from build123d import *

# Parameters (mm, degrees)
F0_R     = 4.8895
F1_DEPTH = 1.5875
F2_R     = 5.08
F3_R     = 5.08
F4_R     = 6.35
F5_R     = 5.08
F7_DEPTH = 12.7
F8_R     = 6.1595
F9_DEPTH = 1.5875
F10_R    = 0.635


with BuildPart() as f1:
    # F0 (on Right) → F1 (new body, symmetric)
    with BuildSketch(Plane.YZ):
        with BuildLine():
            Line((15.980706, -19.05), (23.759998, -9.779))
            ThreePointArc((23.759998, -9.779), (33.538998, 0), (23.759998, 9.779))
            Line((23.759998, 9.779), (15.875, 9.779))
            Line((15.875, 9.779), (10.546717, 3.429))
            Line((10.546717, 3.429), (-10.546717, 3.429))
            Line((-10.546717, 3.429), (-15.875, 9.779))
            Line((-15.875, 9.779), (-23.759998, 9.779))
            ThreePointArc((-23.759998, 9.779), (-33.538998, 0), (-23.759998, -9.779))
            Line((-23.759998, -9.779), (-15.980706, -19.05))
            Line((-15.980706, -19.05), (15.980706, -19.05))
        make_face()
        with Locations((-23.759998, 0)):
            Circle(F0_R, mode=Mode.SUBTRACT)
        with Locations((23.759998, 0)):
            Circle(F0_R, mode=Mode.SUBTRACT)
    extrude(amount=F1_DEPTH, both=True)

    # F2
    f2_edges = [f1.edges().sort_by_distance(p)[0] for p in [
        (0, -15.980706, -19.05),
        (0, 15.980706, -19.05),
    ]]
    fillet(f2_edges, radius=F2_R)

    # F3
    f3_edges = [f1.edges().sort_by_distance(p)[0] for p in [
        (0, -10.546717, 3.429),
        (0, 10.546717, 3.429),
    ]]
    fillet(f3_edges, radius=F3_R)

    # F4
    f4_edges = [f1.edges().sort_by_distance(p)[0] for p in [
        (0, -15.875, 9.779),
        (0, 15.875, 9.779),
    ]]
    fillet(f4_edges, radius=F4_R)

    # F5
    f5_edges = [f1.edges().sort_by_distance(p)[0] for p in [
        (0, -23.759998, -9.779),
        (0, 23.759998, -9.779),
    ]]
    fillet(f5_edges, radius=F5_R)

    # F6 (on Right) → F7 (cut, symmetric)
    with BuildSketch(Plane.YZ):
        with BuildLine():
            Line((10.795, -9.803238), (-10.795, -9.803238))
            ThreePointArc((-10.795, -9.803238), (-13.691762, -12.7), (-10.795, -15.596762))
            Line((-10.795, -15.596762), (10.795, -15.596762))
            ThreePointArc((10.795, -15.596762), (13.691762, -12.7), (10.795, -9.803238))
        make_face()
    extrude(amount=F7_DEPTH, both=True, mode=Mode.SUBTRACT)

    # F8 (on face) → F9 (cut)
    with BuildSketch(Plane.YZ.offset(1.5875)):
        with Locations((-23.759998, 0)):
            Circle(F8_R)
        with Locations((23.759998, 0)):
            Circle(F8_R)
    extrude(amount=-F9_DEPTH, mode=Mode.SUBTRACT)

    # F10
    f10_edges = [f1.edges().sort_by_distance(p)[0] for p in [
        (1.5875, -19.963165, -14.303889),
        (-1.5875, -33.502533, 0.84372),
    ]]
    fillet(f10_edges, radius=F10_R)


solid = f1.part
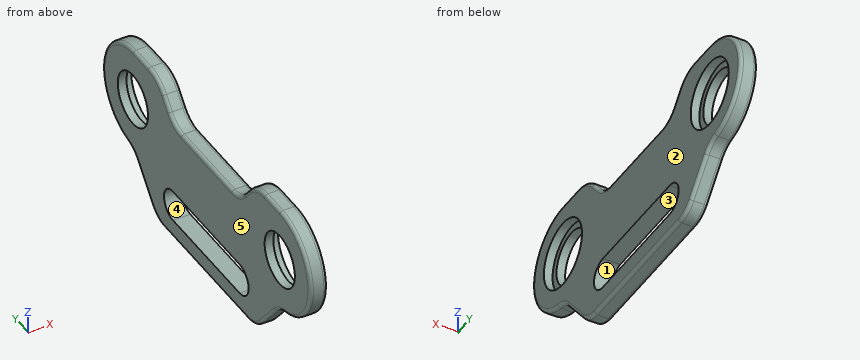
Here's how the part is built. I have some questions about the finished solid (model axes, mm). Face numbers are marked on the shaded views. A direction names the side the tool comes from. Give positions to 0.01 mm unless a question says otherwise; leave off trailing zeros. Loops run counter-clockwise (first coordinate to the right, second up) from the corner with the lowest first, then second, coordinate; pieces in that order, holes last. Notation, with made-up numbers: (68, -1.75) -> (81, -1.75) arc R16 ccw to (81, 28.25) -> close; hole circle Ø3 at (50, 60.5). An arc over 180 degrees is marked (long way). Answer as a JSON object with one key per item and string values. Group by question number.
Item 1: On a 3-axis mill with a long thin cutter (end or side, diameter ignored), from which of +Z, -Z, +X, -X, +Y, -Y can I reach the whole of each face in a straight line? I mean the marked faces 1 and 2. Say none if no direction works.
Item 2: Imagine slicing it at A-A on z = 0. Write out the boundary of the cut face in (x, y) (1 decimal), then the cut area to 3 significant figures.
Item 3: Will these pins go through, and if not, where does the flat tip stop? pin 1 (11 mm diameter, centred on y = 23.76, z = 0, fed in from +X); pin 2 (1.6 mm diameter, centred on x = -0.5, y = -2.5, fed in from +Z).
Item 4: Thinking about a two-plate mould opening in Z: for the marked faces 3, 4 and 5, which applies, pulls with the +Z half, pulls with the -Z half, needs draft (parallel to the pull), parting line crosses it, or undercut?
Item 5: I need wall thicknesses on L1, parallel to Y at x = -0.6, z = 0; L2, parallel to Z at x = 0.35, y = -2; L3, parallel to Y at x = 0.6, z = -5.5. Which ranges of each line are inside material? Lowest first, please.
Answer list:
{
 "1": {"face 1": "+X, -X", "face 2": "+Z, -Z, +X, +Y, -Y"},
 "2": {"outline": "(-1.6, -32.9) arc R0.6 ccw to (-1, -33.5) -> (1, -33.5) arc R0.6 ccw to (1.6, -32.9) -> (1.6, -29.9) -> (0, -29.9) -> (0, -28.6) -> (-1.6, -28.6) -> close; (-1.6, -18.9) -> (0, -18.9) -> (0, -17.6) -> (1.6, -17.6) -> (1.6, 17.6) -> (0, 17.6) -> (0, 18.9) -> (-1.6, 18.9) -> close; (-1.6, 28.6) -> (0, 28.6) -> (0, 29.9) -> (1.6, 29.9) -> (1.6, 32.9) arc R0.6 ccw to (1, 33.5) -> (-1, 33.5) arc R0.6 ccw to (-1.6, 32.9) -> close", "area": "142 mm2"},
 "3": {"pin 1": "stops at x = 0", "pin 2": "stops at z = 3.43"},
 "4": {"face 3": "undercut", "face 4": "undercut", "face 5": "needs draft"},
 "5": {"L1": "y = -33.54 to -28.65, -18.87 to 18.87, 28.65 to 33.54", "L2": "z = -19.05 to -15.6, -9.8 to 3.43", "L3": "y = -31.85 to -26.53, -20.99 to 20.99, 26.53 to 31.85"}
}
